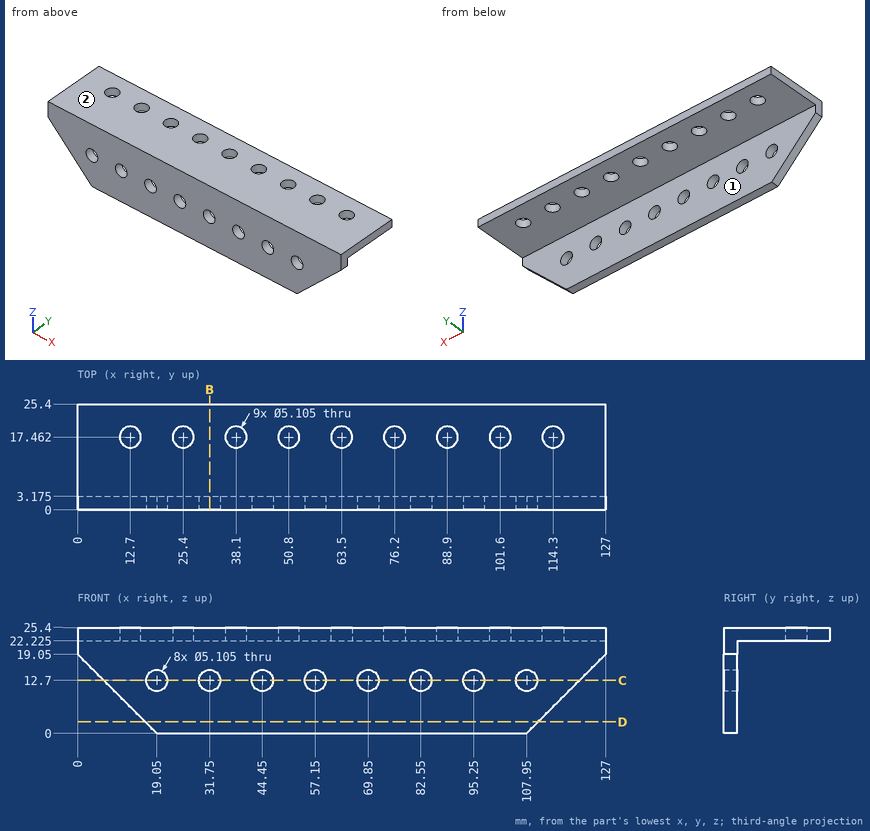
For this review, use the dimensioned drawing (mm, ordinates from the lowest corner) and the shaded views. A direction names the side the tool comes from. Round coordinates to 2 decimals unless told otherwise and drop trailing zeros. Write each loop counter-clockwise with the first axis right and the second up, starting at its lowest first coordinate (ties: lowest second). Pieces come first, ordered by that corner, then holes. Notation, with made-up numbers: (-23.75, -36) - (-16.75, -36) arc R31 cw to (-16.75, -9) - close; hole circle Ø8 at (-15, 46.5). An arc over 180 degrees is marked (long way). Answer as a JSON object with one key per item and string values.
1. For pin 1 Ø6 at (x, y) = (50.8, 17.46) entering from -Z (1 decimal); pin 2 Ø5 at (x, z) = (20, 16.5) entering from +Y (1 decimal), all flat-tipped, find the tip position at first contact; note any pin that passes through.
Response values:
{"pin 1": "stops at z = 22.2", "pin 2": "stops at y = 3.2"}
2. To check wall thickness, follow line 1 along Y through (x, z) = (38.1, 24.3) (1 decimal); line 2 along Z through (x, y) = (35, 12.5) (1 decimal); line 3 along Y through (x, z) = (28, 5) (1 decimal). State the ranges of each line that lie inside material, in increasing order.
Response values:
{"line 1": "y = 0 to 14.9, 20 to 25.4", "line 2": "z = 22.2 to 25.4", "line 3": "y = 0 to 3.2"}
3. We need section B-B on x = 31.75. Give the boundary of the cut face in (y, z) (1 decimal).
Response values:
{"outline": "(0, 0) - (3.2, 0) - (3.2, 10.1) - (0, 10.1) - close; (0, 15.3) - (3.2, 15.3) - (3.2, 22.2) - (25.4, 22.2) - (25.4, 25.4) - (0, 25.4) - close"}
4. Tool access review of the marked faces 1 and 2: name each direction out of +Z, -Z, +X, -X, +Y, -Y from which nothing blocks a thin tool from reaching the whole face with its end or side.
Response values:
{"face 1": "-Z, +X, -X, +Y", "face 2": "+Z, +X, -X, +Y, -Y"}
5. We need section C-C on z = 12.7. Count the separate pieces of the cut face and the enclosed holes in it, then the cut area to 3 significant figures.
Response values:
{"separate pieces": "9", "enclosed holes": "0", "area": "233 mm2"}
6. We need section D-D on z = 2.75. Give the boundary of the cut face in (x, y) (1 decimal).
Response values:
{"outline": "(16.3, 0) - (110.7, 0) - (110.7, 3.2) - (16.3, 3.2) - close"}
